Study the drawing (mm; zero at the part's minimum x, y, z) and answer. A direction names the side the tool comes from. Coordinates: 2 decimals unless noted, no trailing zeros. Write each loop counter-clockwise with the first axis right and the second up, starting at its lowest first coordinate (ties: lowest second). Pieces come first, ordered by that corner, then holes. Notation, with made-up numbers: M -40,-37.5 L 19,-37.5 A6 cw 19,-32.5 Z; hole C 70.5,64 d11. An arc over 180 degrees is marked long. Answer as a JSON object with one key per item and string values. Group by question number.
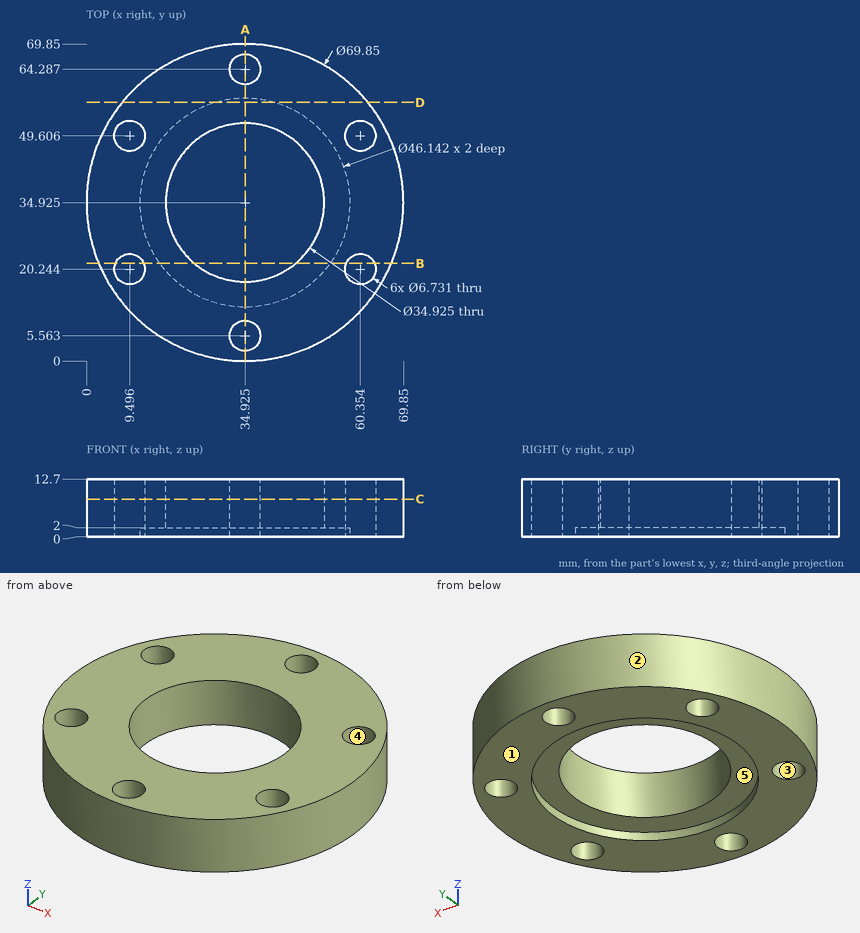
Item 1: A cutting plane is placed at A-A, the plane x = 35. Write down the section's boundary in (y, z).
Item 2: A cutting plane is placed at B-B, the plane y = 21.5. Write down the section's boundary in (x, z) (1 decimal).
Item 3: A cutting plane is placed at C-C, the plane z = 8.25. State how many separate pieces and enclosed holes the cut face has, and give its area (3 significant figures).
Item 4: A tool of negligible diameter and unlimited length cuts with its end or side. For the marked faces 4 and 5, from which of +Z, -Z, +X, -X, +Y, -Y can it reach the whole face along a straight path? Write none if from no direction.
Item 5: A cutting plane is placed at D-D, the plane y = 57. Write down the section's boundary in (x, z).
Item 6: Flat-ended cylindrical pins translate along their axes: pin 1 Ø2 at (x, z) = (45.5, 11) entering from +Y; pin 2 Ø5 at (y, z) = (17.5, 2) entering from -X; pin 3 Ø6 at (x, y) = (34.92, 64.29) entering from +Z; pin 4 Ø1.5 at (x, z) = (57, 8) entering from +Y (1 decimal). Find the tip coordinate at first contact, or state that the pin passes through.
Item 7: For a pull along X with two mould halves and no side action, classify the marked faces 1, 2 and 3 as +X half, -X half, draft (parallel to the pull), parting line (faces both ways), or undercut.
Item 8: Consider L1, parallel to Y at x = 9.5, z = 7.5; L2, parallel to Y at x = 37, z = 11.5 (1 decimal); L3, parallel to Y at x = 10, z = 3.25 (1 decimal). Determine where each line is inside the solid, lowest interval first. Write a range as from..to.
Answer:
{
 "1": {"outline": "M 0,0 L 2.2,0 L 2.2,12.7 L 0,12.7 Z; M 8.93,0 L 11.85,0 L 11.85,2 L 17.46,2 L 17.46,12.7 L 8.93,12.7 Z; M 52.39,2 L 58,2 L 58,0 L 60.92,0 L 60.92,12.7 L 52.39,12.7 Z; M 67.65,0 L 69.85,0 L 69.85,12.7 L 67.65,12.7 Z"},
 "2": {"outline": "M 2.7,0 L 6.4,0 L 6.4,12.7 L 2.7,12.7 Z; M 12.6,0 L 16.2,0 L 16.2,2 L 23.8,2 L 23.8,12.7 L 12.6,12.7 Z; M 46.1,2 L 53.7,2 L 53.7,0 L 57.2,0 L 57.2,12.7 L 46.1,12.7 Z; M 63.5,0 L 67.2,0 L 67.2,12.7 L 63.5,12.7 Z"},
 "3": {"separate pieces": "1", "enclosed holes": "7", "area": "2,660 mm2"},
 "4": {"face 4": "+Z, -Z", "face 5": "-Z"},
 "5": {"outline": "M 7.86,0 L 28.22,0 L 28.22,2 L 41.63,2 L 41.63,0 L 61.99,0 L 61.99,12.7 L 7.86,12.7 Z"},
 "6": {"pin 1": "y = 68.51", "pin 2": "x = 3.35", "pin 3": "through", "pin 4": "y = 62.6"},
 "7": {"face 1": "draft", "face 2": "parting line", "face 3": "undercut"},
 "8": {"L1": "10.98..16.88, 23.61..46.24, 52.97..58.87", "L2": "0.1..2.9, 8.2..17.6, 52.3..61.6, 66.9..69.8", "L3": "10.5..16.9, 23.6..46.3, 52.9..59.4"}
}
